from build123d import *

# Parameters (mm, degrees)
EXTRUDE1_DEPTH      = 75
EXTRUDE1_DEPTH_BACK = 75
FILLET2_R           = 5


with BuildPart() as part:
    # Sketch1 → Extrude1 (new, two sides: drawn at the far end of the back side and taken through both)
    with BuildSketch(Plane.XY.offset(-EXTRUDE1_DEPTH_BACK)):
        with BuildLine():
            Line((68, -58), (75, -58))
            Line((75, -58), (75, -80))
            Line((75, -80), (-75, -80))
            Line((-75, -80), (-75, -5))
            Line((-75, -5), (-68, -5))
            add(Edge.make_bspline(
                [(-68, -5), (19.719434236, -5), (-30.32506556, -58), (68, -58)],
                knots=[0, 0, 0, 0, 1, 1, 1, 1], degree=3))
        make_face()
    extrude(amount=EXTRUDE1_DEPTH + EXTRUDE1_DEPTH_BACK)

    # Sketch2 → Revolve1 (revolve)
    with BuildSketch(Plane.XY):
        with BuildLine():
            Line((0, -60), (60, -60))
            ThreePointArc((60, -60), (42.426406871, -17.573593129), (0, 0))
            Line((0, 0), (0, -60))
        make_face()
    revolve(axis=Axis((0, 11.185160428, 0), (0, -1, 0)))

    # Fillet2
    fillet2_edges = [part.edges().sort_by_distance(p)[0] for p in [
        (9.137379972, -44.707678169, -57.294442834),
    ]]
    fillet(fillet2_edges, radius=FILLET2_R)


solid = part.part
Verification items for the finished model (mm, model axes). A direction names the side the tool comes from. Round coordinates to 2 decimals unless told otherwise and drop trailing zeros.
(1) Material ranges on line 1 (Z direction, x = 19, y = -33); line 2 (Y direction, x = 29, z = 4); line 3 (Z direction, x = 41.5, y = -53), recorded low to high.
Returned:
line 1: z = -50.1 to 50.1
line 2: y = -80 to -7.63
line 3: z = -42.82 to 42.82
(2) Depth check by flat-ended pin: pin 1 Ø6 at (y, z) = (-50, -12.5) entering from +X; pin 2 Ø2 at (x, z) = (-70, 37) entering from +Y; pin 3 Ø3.5 at (x, z) = (71.5, 13.5) entering from +Y. Enter the tip coordinate at first touch or a pass-through.
Returned:
pin 1: stops at x = 58.57
pin 2: stops at y = -5
pin 3: stops at y = -58
(3) Access from +Z, -Z, +X, -X, +Y, -Y to the whole of each face (thin tool, end or side, straight path). Record for faces 1 (the flat face through (75, -69, -1)), 2 (the flat face through (71, -58, -1)), 3 (the flat face through (-72, -5, -1)).
Returned:
face 1: +Z, -Z, +X, +Y, -Y
face 2: +Z, -Z, +X, +Y
face 3: +Z, -Z, -X, +Y
